For this review, use the dimensioned drawing (mm, ordinates from the lowest corner) and the shaded views. A direction names the side the tool comes from. Give positions to 0.01 mm unless a question says otherwise; leave off trailing zeros. Order: outer loops, then holes, each group sorted by start corner. A loop starts at its lowest first (then second) coordinate and runs counter-clockwise, first axis right, second up. Notation, with made-up numbers: (45.25, -26) - (54.25, -26) arc R29 cw to (54.25, 6) - close; hole circle Ø9 at (75, -10.5). An arc over 180 degrees is marked (long way). One line per item, written item: value.
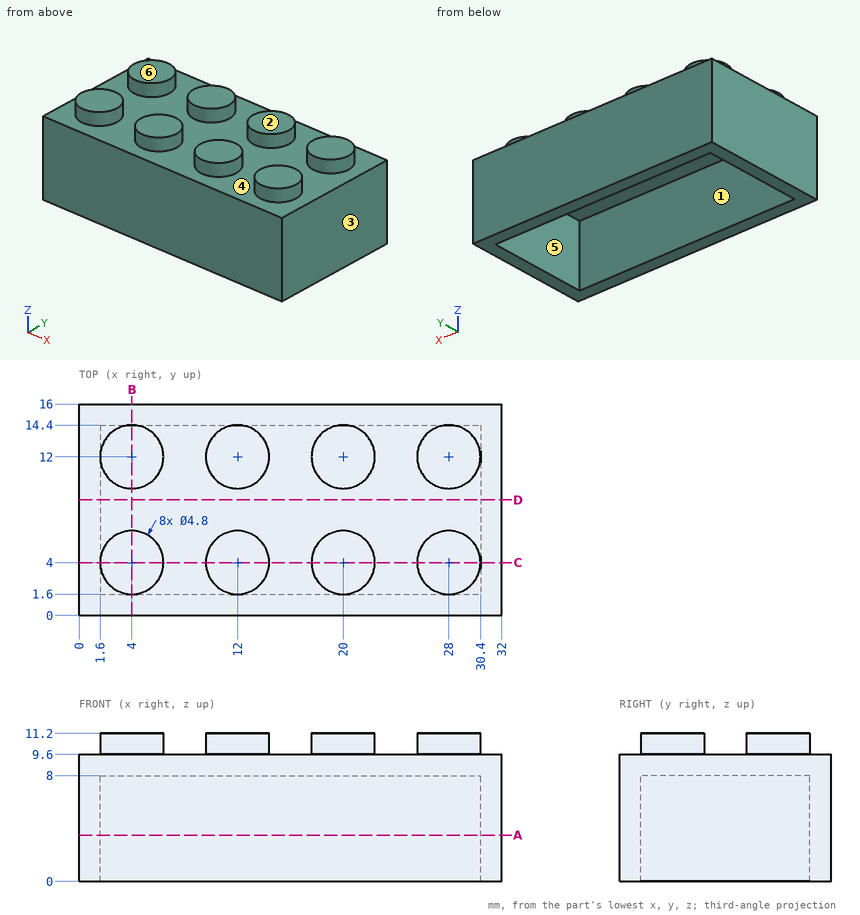
(1) Take a section at D-D (y = 8.75). Write out the cut boundary in (x, z), then the cut area to 3 significant figures.
Answers below:
outline: (0, 0) - (1.6, 0) - (1.6, 8) - (30.4, 8) - (30.4, 0) - (32, 0) - (32, 9.6) - (0, 9.6) - close
area: 76.8 mm^2
(2) Take a section at B-B (x = 4). Write out the cut boundary in (y, z).
Answers below:
outline: (0, 0) - (1.6, 0) - (1.6, 8) - (14.4, 8) - (14.4, 0) - (16, 0) - (16, 9.6) - (14.4, 9.6) - (14.4, 11.2) - (9.6, 11.2) - (9.6, 9.6) - (6.4, 9.6) - (6.4, 11.2) - (1.6, 11.2) - (1.6, 9.6) - (0, 9.6) - close
(3) Wall thickness on line 1 (X direction, y = 11.25, z = 3.5); line 2 (Y direction, x = 20.5, z = 4); line 3 (X direction, y = 3.5, z = 10): over which ranges is each line inside the solid? List them lowest first. Write a range as from..to.
Answers below:
line 1: x = 0..1.6, 30.4..32
line 2: y = 0..1.6, 14.4..16
line 3: x = 1.65..6.35, 9.65..14.35, 17.65..22.35, 25.65..30.35
(4) For P1, Ø2.5, axis at y = 6.5, z = 3.5, coming from the -X side; P2, Ø6.5, axis at x = 14, y = 6.5, coming from the -Z side, all flat-tipped, find the tip position at first contact; note any pin that passes through.
Answers below:
P1: stops at x = 0
P2: stops at z = 8
(5) Take a section at A-A (z = 3.5). Write out the cut boundary in (x, y).
Answers below:
outline: (0, 0) - (32, 0) - (32, 16) - (0, 16) - close; hole (1.6, 1.6) - (30.4, 1.6) - (30.4, 14.4) - (1.6, 14.4) - close
(6) Take a section at C-C (y = 4). Write out the cut boundary in (x, z), then the cut area to 3 significant figures.
Answers below:
outline: (0, 0) - (1.6, 0) - (1.6, 8) - (30.4, 8) - (30.4, 0) - (32, 0) - (32, 9.6) - (30.4, 9.6) - (30.4, 11.2) - (25.6, 11.2) - (25.6, 9.6) - (22.4, 9.6) - (22.4, 11.2) - (17.6, 11.2) - (17.6, 9.6) - (14.4, 9.6) - (14.4, 11.2) - (9.6, 11.2) - (9.6, 9.6) - (6.4, 9.6) - (6.4, 11.2) - (1.6, 11.2) - (1.6, 9.6) - (0, 9.6) - close
area: 108 mm^2
(7) Machinability: for the marked faces 4, 5 and 6, which of the approach directions +Z, -Z, +X, -X, +Y, -Y give a long, thin tool a straight path to every point of the face, cutting with its end or side? Answer none if there is none.
Answers below:
face 4: +Z
face 5: -Z
face 6: +Z, +X, -X, +Y, -Y
(8) Draft analysis for pull direction X (two halves, no side actions). For the marked faces 1, 2 and 3, state which applies: pulls with the +X half, pulls with the -X half, needs draft (parallel to the pull), parting line crosses it, or undercut.
Answers below:
face 1: undercut
face 2: needs draft
face 3: pulls with the +X half
